from build123d import *

# Parameters (mm, degrees)
F1_DEPTH = 2
F3_DEPTH = 2
F4_R     = 2.5
F5_DEPTH = 4.001


with BuildPart() as f1:
    # F0 (on Top) → F1 (new body)
    with BuildSketch(Plane.XY):
        with BuildLine():
            ThreePointArc((20.499703, 0.052712), (18.867793, 3.902856), (15.000031, 5.492559))
            Line((15.000031, 5.492559), (-14.999969, 5.492559))
            ThreePointArc((-14.999969, 5.492559), (-18.889056, 3.881647), (-20.499969, -0.007441))
            ThreePointArc((-20.499969, -0.007441), (-18.889056, -3.896528), (-14.999969, -5.507441))
            Line((-14.999969, -5.507441), (15.000031, -5.507441))
            ThreePointArc((15.000031, -5.507441), (18.910328, -3.875202), (20.499703, 0.052712))
        make_face()
    extrude(amount=F1_DEPTH)

    # F2 (on face) → F3 (join)
    with BuildSketch(Plane(origin=(0, 0, 0), x_dir=(1, 0, 0), z_dir=(0, 0, -1))):
        with BuildLine():
            Line((14.637494, 3.734077), (-14.637494, 3.734077))
            ThreePointArc((-14.637494, 3.734077), (-18.732699, 0), (-14.637494, -3.734077))
            Line((-14.637494, -3.734077), (14.637494, -3.734077))
            ThreePointArc((14.637494, -3.734077), (18.732699, 0), (14.637494, 3.734077))
        make_face()
    extrude(amount=F3_DEPTH)

    # F4 (on face) → F5 (cut, through all)
    with BuildSketch(Plane.XY.offset(2)):
        with Locations((-14.999969, -0.007441)):
            Circle(F4_R)
        with Locations((15.000031, -0.007441)):
            Circle(F4_R)
    extrude(amount=-F5_DEPTH, mode=Mode.SUBTRACT)


solid = f1.part
Build history of the part. All positions in model axes, mm. A direction names the side the tool comes from. Give positions to 0.01 mm unless a question says otherwise; leave off trailing zeros. Write each loop counter-clockwise with the first axis right and the second up, starting at its lowest first coordinate (ties: lowest second). Pieces come first, ordered by that corner, then holes. Notation, with made-up numbers: (26.5, 39.25) - (67.5, 39.25) arc R20 cw to (67.5, 55.25) - close; hole circle Ø6 at (40.5, -16.75). An arc over 180 degrees is marked (long way). Use one line per item in the form item = value. Start each with the question number.
1. Probe line 1 (Z direction, x = -6, y = 4.75); line 2 (Y direction, x = -7, z = -1.2); line 3 (X direction, y = 0.5, z = 0.35). List the from-to ranges inside material, lowest first. Write a range as [from, to].
2. Band-saw the part on C-C on y = 3. Write the cut outline in (x, z).
3. Drop flat-ended pins along their axis: pin 1 Ø2 at (x, z) = (-15.5, 0) entering from -Y; pin 2 Ø1 at (y, z) = (-1, 0) entering from +X; pin 3 Ø0.6 at (x, z) = (2.5, -0.5) entering from +Y; pin 4 Ø0.6 at (x, z) = (6, -1) entering from -Y. Give the stop position or say it passes through.
4. Band-saw the part on B-B on x = 14. Write the cut outline in (y, z), plus the area to 3 significant figures.
5. Band-saw the part on D-D on x = -17. Write the cut outline in (y, z).
6. Two-plate mould, pull along Y, no slides. Class faces 3 (the face through (0, -5.507, 1)), 4 (the face through (-18.73, -0.09, -0.99)), 5 (the face through (17.31, -0.96, 0.03)): released by +Y, released by -Y, zero draft, split by the parting line, or undercut.
7. Band-saw the part on A-A on z = 0.55. Write the cut outline in (x, y), plus the area to 3 significant figures.
8. 3-axis set-ups, long thin cutter, end or side, ignore diameter. For faces 1 (the face through (0, 4, 0)), 2 (the face through (0, 5.493, 1)): which of +Z, -Z, +X, -X, +Y, -Y reach the whole face in a straight line?
Conclusion:
q1.line_1 = [0, 2]
q1.line_2 = [-3.73, 3.73]
q1.line_3 = [-20.48, -17.45], [-12.55, 12.55], [17.45, 20.48]
q2.outline = (-19.6, 0) - (-17.23, 0) - (-17.23, -2) - (17.23, -2) - (17.23, 0) - (19.6, 0) - (19.6, 2) - (-19.6, 2) - close
q3.pin_1 = -5.51
q3.pin_2 = 20.48
q3.pin_3 = 3.73
q3.pin_4 = -3.73
q4.outline = (-5.51, 0) - (-3.73, 0) - (-3.73, -2) - (-2.3, -2) - (-2.3, 2) - (-5.51, 2) - close; (2.28, -2) - (3.73, -2) - (3.73, 0) - (5.49, 0) - (5.49, 2) - (2.28, 2) - close
q4.area = 18.6 mm²
q5.outline = (-5.13, 0) - (-3.16, 0) - (-3.16, -2) - (-1.51, -2) - (-1.51, 2) - (-5.13, 2) - close; (1.49, -2) - (3.16, -2) - (3.16, 0) - (5.12, 0) - (5.12, 2) - (1.49, 2) - close
q6.face_3 = released by -Y
q6.face_4 = split by the parting line
q6.face_5 = undercut
q7.outline = (-20.5, -0.01) arc R5.5 ccw to (-15, -5.51) - (15, -5.51) arc R5.5 ccw to (20.5, 0.05) arc R5.5 ccw to (15, 5.49) - (-15, 5.49) arc R5.5 ccw to start; hole circle Ø5 at (-15, -0.01); hole circle Ø5 at (15, -0.01)
q7.area = 386 mm²
q8.face_1 = -Z
q8.face_2 = +Z, -Z, +X, -X, +Y
